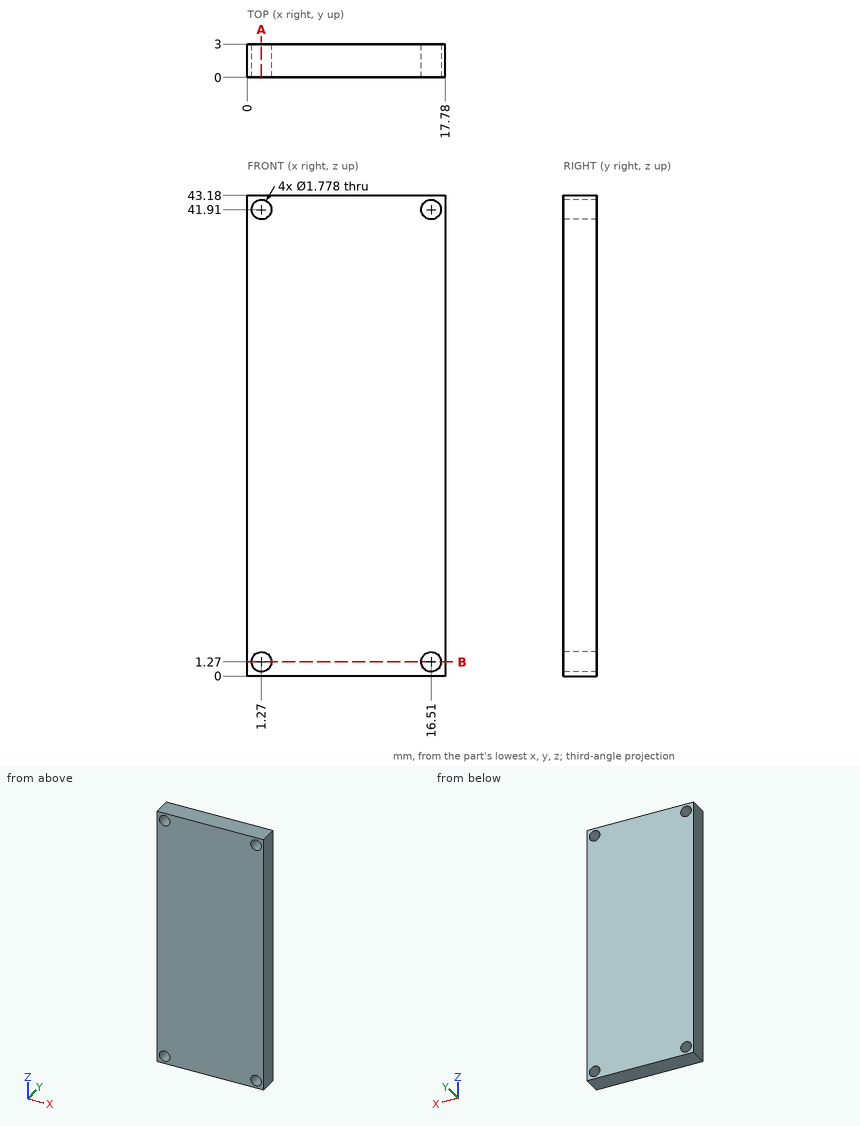
The drawing under review shows one solid part. Ordinate dimensions are in mm from its lowest x, y, z. Give positions to 0.01 mm unless a question says otherwise; leave off trailing zeros. Write each loop counter-clockwise with the first axis right and the second up, starting at its lowest first coordinate (ties: lowest second). Pieces come first, ordered by that corner, then holes. Notation, with made-up numbers: (76.25, 63) - (88.25, 63) arc R9 cw to (88.25, 76) - close; hole circle Ø4 at (28.25, -14.5). An arc over 180 degrees is marked (long way). Answer in a Markdown table with one row per item. Add a question column.
1. We need section B-B on z = 1.27. Write out the cut boundary in (x, y), then the cut area to 3 significant figures.
2. We need section A-A on x = 1.27. Write out the cut boundary in (y, z), then the cut area to 3 significant figures.
3. Wall thickness on line 1 along Z through (x, y) = (16.51, 1.55); line 2 along X through (y, z) = (1.55, 41.91): over which ranges is each line inside the solid? List them lowest first. Write a range as [from, to].
Ans:
| question | item | result |
|---|---|---|
| 1 | outline | (0, 0) - (0.38, 0) - (0.38, 3) - (0, 3) - close; (2.16, 0) - (15.62, 0) - (15.62, 3) - (2.16, 3) - close; (17.4, 0) - (17.78, 0) - (17.78, 3) - (17.4, 3) - close |
| 1 | area | 42.7 mm^2 |
| 2 | outline | (0, 0) - (3, 0) - (3, 0.38) - (0, 0.38) - close; (0, 2.16) - (3, 2.16) - (3, 41.02) - (0, 41.02) - close; (0, 42.8) - (3, 42.8) - (3, 43.18) - (0, 43.18) - close |
| 2 | area | 119 mm^2 |
| 3 | line 1 | z = [0, 0.38], [2.16, 41.02], [42.8, 43.18] |
| 3 | line 2 | x = [0, 0.38], [2.16, 15.62], [17.4, 17.78] |
